Autodesk Inventor part; units mm, degrees
ref_plane "YZ Plane" through (0, 0, 0) normal (1, 0, 0) x (0, 1, 0)
ref_plane "XZ Plane" through (0, 0, 0) normal (0, 1, 0) x (-1, 0, 0)
ref_plane "XY Plane" through (0, 0, 0) normal (0, 0, 1) x (1, 0, 0)
sketch "Skizze1" plane through (0, 0, 0) normal (0, 0, 1) x (1, 0, 0)
  line L0 (-8.4, 11.4) -> (8.4, 11.4)
  line L1 (8.4, 11.4) -> (8.4, -11.4)
  line L2 (8.4, -11.4) -> (-8.4, -11.4)
  line L3 (-8.4, -11.4) -> (-8.4, 11.4)
  line L4 (-13.6739, 0) -> (13.6739, 0)
  line L5 (0, -25.1399) -> (0, 25.1399)
  line L6 (-7.35, 9.75) -> (7.35, 9.75)
  line L7 (7.35, 9.75) -> (7.35, -9.75)
  line L8 (7.35, -9.75) -> (-7.35, -9.75)
  line L9 (-7.35, -9.75) -> (-7.35, 9.75)
  line L10 (-8.56, 17.75) -> (8.56, 17.75)
  line L11 (9.56, 16.75) -> (9.56, -16.75)
  line L12 (8.56, -17.75) -> (-8.56, -17.75)
  line L13 (-9.56, -16.75) -> (-9.56, 16.75)
  circle A0 centre (0, 14.45) radius 1.6
  line L14 (-9.56, -17.75) -> (9.56, -17.75)
  circle A1 centre (0, -14.45) radius 1.6
  arc A2 (-8.56, 17.75) -> (-9.56, 16.75) centre (-8.56, 16.75) ccw
  arc A3 (9.56, 16.75) -> (8.56, 17.75) centre (8.56, 16.75) ccw
  arc A4 (8.56, -17.75) -> (9.56, -16.75) centre (8.56, -16.75) ccw
  arc A5 (-9.56, -16.75) -> (-8.56, -17.75) centre (-8.56, -16.75) ccw
  line L15 (7.35, -6.55) -> (-7.35, -6.55)
  point P0 (0, 0)
  point P1 (-9.56, 17.75)
  point P2 (9.56, 17.75)
  dimension "d0" = 16.8
  dimension "d1" = 22.8
  dimension "d2" = 19.5
  dimension "d3" = 14.7
  dimension "d4" = 35.5
  dimension "d5" = 19.12
  dimension "d6" = 3.2
  dimension "d7" = 28.9
  dimension "d8" = 1
  dimension "d14" = 3.2
extrude "Extrusion1" add sketch "Skizze1" against normal blind 7.3 contours L0 L5 L6 L9 L4 L3 | L0 L1 L4 L7 L6 L5 | L4 L9 L8 L5 L2 L3 | L1 L2 L5 L8 L7 L4
extrude "Extrusion2" add sketch "Skizze1" along normal blind 2.5 contours L3 L4 L13 A2 L10 L5 A0 L0 | L0 L5 L6 L9 L4 L3 | L5 A0 L10 A3 L11 L4 L1 L0 | L0 L1 L4 L7 L6 L5 | L4 L9 L8 L5 L2 L3 | L3 L2 L5 A1 L12 A5 L13 L4 | L4 L11 A4 L12 L5 A1 L2 L1 | L1 L2 L5 L8 L7 L4
extrude "Extrusion3" add sketch "Skizze1" against normal blind 1 from surface at 2.5 contours L15 L5 L8 L9 | L15 L7 L8 L5
fillet "Rundung1" radius 0.5 10 edges at (-9.2671, 17.4571, 2.5) (-9.56, 0, 2.5) (-9.2671, -17.4571, 2.5) (0, -17.75, 2.5) (9.2671, -17.4571, 2.5) (9.56, 0, 2.5) (9.2671, 17.4571, 2.5) (0, 17.75, 2.5) (-1.6, 14.45, 2.5) (-1.6, -14.45, 2.5)
properties part number "Delock_86213_Grob"
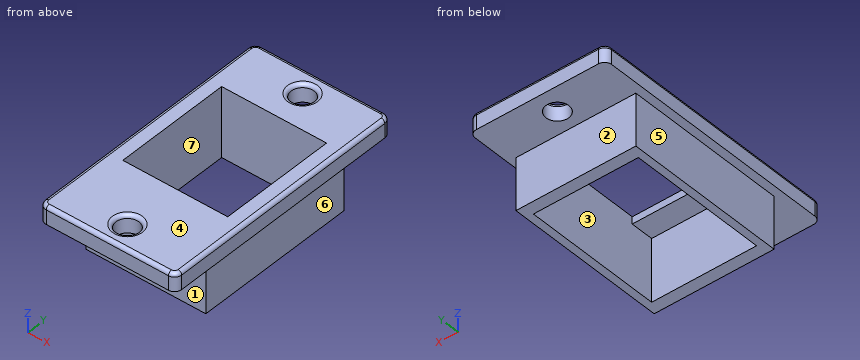
Model file for the job. Use its own axes, mm. Face numbers are marked on the shaded views. A direction names the side the tool comes from. Coordinates: 2 decimals unless noted, no trailing zeros. Order: outer loops, then holes, each group sorted by start corner. A loop starts at its lowest first (then second) coordinate and runs counter-clockwise, first axis right, second up. Notation, with made-up numbers: (75, -7) -> (129, -7) arc R19 ccw to (129, 0) -> close; hole circle Ø8 at (22, 49). An arc over 180 degrees is marked (long way). Answer as a JSON object with one key per item and string values. Group by question number.
1) Cut at A-A, the plane y = -4. Write the cut outline in (x, z).
2) Cut at C-C, the plane x = 0. Write the cut outline in (y, z), then the cut area to 3 significant figures.
3) Pull direction Y, two halves, no side cores. Call the marked faces 1, 2, 3 and 4: +Y half, -Y half, draft (parallel to the pull), parting line (faces both ways), or undercut.
4) Which spindle directions (+Z, -Z, +X, -X, +Y, -Y) get a long thin tool onto all of the face, cutting with end or side? Do the marked faces 5, 6 and 7. Say none if no direction does.
5) Drill centre lines: L1, parallel to Y at x = 0, z = 0.4; L2, parallel to Y at x = 2.25, z = -3; L3, parallel to X at y = 3, z = -7. Where is each one in solid material? Low to high.
6) Cut at B-B, the plane z = -2. Write the cut outline in (x, y).
7) Flat gauge pins, fed straight in: pin 1 (3.5 mm diameter, centred on y = 4.5, z = -2, fed in from +X); pin 2 (5 mm diameter, centred on y = -2.5, z = -6, fed in from -X); pin 3 (1.5 mm diameter, centred on x = 5, z = -1, fed in from +Y). Where does each tip first touch, or does it go through?
8) Cut at D-D, the plane x = -3.75. Write the cut outline in (y, z).
Check values:
{
 "1": {"outline": "(-9.56, 0) -> (-8.4, 0) -> (-8.4, -7.3) -> (-7.35, -7.3) -> (-7.35, 2.5) -> (-9.06, 2.5) arc R0.5 ccw to (-9.56, 2) -> close; (7.35, -7.3) -> (8.4, -7.3) -> (8.4, 0) -> (9.56, 0) -> (9.56, 2) arc R0.5 ccw to (9.06, 2.5) -> (7.35, 2.5) -> close"},
 "2": {"outline": "(-17.75, 0) -> (-16.05, 0) -> (-16.05, 2) arc R0.5 ccw to (-16.55, 2.5) -> (-17.25, 2.5) arc R0.5 ccw to (-17.75, 2) -> close; (-12.85, 0) -> (-11.4, 0) -> (-11.4, -7.3) -> (-9.75, -7.3) -> (-9.75, 1.5) -> (-6.55, 1.5) -> (-6.55, 2.5) -> (-12.35, 2.5) arc R0.5 ccw to (-12.85, 2) -> close; (9.75, -7.3) -> (11.4, -7.3) -> (11.4, 0) -> (12.85, 0) -> (12.85, 2) arc R0.5 ccw to (12.35, 2.5) -> (9.75, 2.5) -> close; (16.05, 0) -> (17.75, 0) -> (17.75, 2) arc R0.5 ccw to (17.25, 2.5) -> (16.55, 2.5) arc R0.5 ccw to (16.05, 2) -> close", "area": "51.0 mm²"},
 "3": {"face 1": "-Y half", "face 2": "+Y half", "face 3": "undercut", "face 4": "draft"},
 "4": {"face 5": "-Z, -X, +Y, -Y", "face 6": "-Z, +X, +Y, -Y", "face 7": "-Z"},
 "5": {"L1": "y = -17.75 to -16.05, -12.85 to -9.75, 9.75 to 12.85, 16.05 to 17.75", "L2": "y = -11.4 to -9.75, 9.75 to 11.4", "L3": "x = -8.4 to -7.35, 7.35 to 8.4"},
 "6": {"outline": "(-8.4, -11.4) -> (8.4, -11.4) -> (8.4, 11.4) -> (-8.4, 11.4) -> close; hole (-7.35, -9.75) -> (7.35, -9.75) -> (7.35, 9.75) -> (-7.35, 9.75) -> close"},
 "7": {"pin 1": "stops at x = 8.4", "pin 2": "stops at x = -8.4", "pin 3": "stops at y = 11.4"},
 "8": {"outline": "(-17.75, 0) -> (-11.4, 0) -> (-11.4, -7.3) -> (-9.75, -7.3) -> (-9.75, 1.5) -> (-6.55, 1.5) -> (-6.55, 2.5) -> (-17.25, 2.5) arc R0.5 ccw to (-17.75, 2) -> close; (9.75, -7.3) -> (11.4, -7.3) -> (11.4, 0) -> (17.75, 0) -> (17.75, 2) arc R0.5 ccw to (17.25, 2.5) -> (9.75, 2.5) -> close"}
}
